Verification items for the finished model (mm, model axes). A direction names the side the tool comes from. Give positions to 0.01 mm unless a question says otherwise; leave off trailing zeros. Order: outer loops, then holes, each group sorted by start corner. A loop starts at its lowest first (then second) coordinate and runs counter-clockwise, first axis right, second up.
from build123d import *

# Parameters (mm, degrees)
F0_W     = 152.4
F0_H     = 152.4
F1_DEPTH = 6.35
F2_R     = 19.05
F3_DEPTH = 6.351
F4_R     = 3.175
F5_DEPTH = 5.08
F6_W     = 144.78
F6_H     = 7.62
F7_DEPTH = 25.4


with BuildPart() as f1:
    # F0 (on Front) → F1 (new body)
    with BuildSketch(Plane.XZ):
        Polygon((76.2, 76.2), (0, 0), (152.4, 0), align=None)
        with Locations((76.2, -76.2)):
            Rectangle(F0_W, F0_H)
    extrude(amount=F1_DEPTH)

    # F2 (on face) → F3 (cut, through all)
    with BuildSketch(Plane.XZ.offset(6.35)):
        with Locations((76.2, -76.2)):
            Circle(F2_R)
    extrude(amount=-F3_DEPTH, mode=Mode.SUBTRACT)

    # F4 (on face) → F5 (cut)
    with BuildSketch(Plane.XZ.offset(6.35)):
        with Locations((76.2, -102.87)):
            Circle(F4_R)
    extrude(amount=-F5_DEPTH, mode=Mode.SUBTRACT)

    # F6 (on face) → F7 (cut)
    with BuildSketch(Plane.XZ.offset(6.35)):
        with Locations((76.2, -142.24)):
            Rectangle(F6_W, F6_H)
    extrude(amount=-F7_DEPTH, mode=Mode.SUBTRACT)


solid = f1.part
(1) Scan lines: line 1 (Z direction, x = 76.2, y = -4.35) (3 decimals); line 2 (Z direction, x = 83.5, y = -4); line 3 (Z direction, x = 93, y = -3). Record each from-to range of solid material in increasing order.
Solved:
line 1: z = -152.4 to -146.05, -138.43 to -106.045, -99.695 to -95.25, -57.15 to 76.2
line 2: z = -152.4 to -146.05, -138.43 to -93.8, -58.6 to 68.9
line 3: z = -152.4 to -146.05, -138.43 to -85.18, -67.22 to 59.4
(2) Section check D-D, the plane x = 89. Enter the section's corners in (y, z).
Solved:
outline: (-6.35, -152.4) - (0, -152.4) - (0, -146.05) - (-6.35, -146.05) - close; (-6.35, -138.43) - (0, -138.43) - (0, -90.31) - (-6.35, -90.31) - close; (-6.35, -62.09) - (0, -62.09) - (0, 63.4) - (-6.35, 63.4) - close
(3) Set-up check for faces 1 (the cylindrical face through (75.51, -3.85, -105.97)), 2 (the flat face through (39, -3, 39)), 3 (the flat face through (75, -3, -146.05)): record each of +Z, -Z, +X, -X, +Y, -Y from which the full face is reachable in a straight line by a thin tool's end or side.
Solved:
face 1: -Y
face 2: +Z, -X, +Y, -Y
face 3: +Y, -Y
(4) Section check A-A, the plane z = -76.2. Enter the section's corners in (x, y).
Solved:
outline: (0, -6.35) - (57.15, -6.35) - (57.15, 0) - (0, 0) - close; (95.25, -6.35) - (152.4, -6.35) - (152.4, 0) - (95.25, 0) - close
(5) Section check C-C, the plane y = -4.5. Enter the section's corners in (x, z) (3 decimals), then the cut area to 3 significant figures.
Solved:
outline: (0, -152.4) - (152.4, -152.4) - (152.4, 0) - (76.2, 76.2) - (0, 0) - close; hole (3.81, -146.05) - (148.59, -146.05) - (148.59, -138.43) - (3.81, -138.43) - close; hole circle Ø38.1 at (76.2, -76.2); hole circle Ø6.35 at (76.2, -102.87)
area: 26,800 mm2
(6) Release check for a two-part mould opening along Z. For faces 4 (the flat face through (3.81, -3, -142)), 5 (the flat face through (75, -3, -152.4)), 6 (the flat face through (114.8, -3.1, 37.6)) record: pulls with the +Z half, pulls with the -Z half, needs draft (parallel to the pull), parting line crosses it, or undercut.
Solved:
face 4: undercut
face 5: pulls with the -Z half
face 6: pulls with the +Z half
(7) Go/stop test with flat-tipped pins: pin 1 (2 mm diameter, centred on y = -2, z = -73.5, fed in from -X); pin 2 (5.5 mm diameter, centred on x = 76.2, z = -102.87, fed in from -Y); pin 3 (3 mm diameter, centred on x = 82, y = -3.5, fed in from +Z); pin 4 (1.5 mm diameter, centred on x = 107.5, y = -2, fed in from +Z). Record where each tip stops, or that it passes through.
Solved:
pin 1: stops at x = 0
pin 2: stops at y = -1.27
pin 3: stops at z = 71.9
pin 4: stops at z = 45.65
(8) Section check B-B, the plane x = 112. Enter the section's corners in (y, z).
Solved:
outline: (-6.35, -152.4) - (0, -152.4) - (0, -146.05) - (-6.35, -146.05) - close; (-6.35, -138.43) - (0, -138.43) - (0, 40.4) - (-6.35, 40.4) - close
